```python
from build123d import *

# Parameters (mm, degrees)
EXTRUDE_1_DEPTH     = 4
CUT_EXTRUDE_1_DEPTH = 1
FILLET_1_R          = 1
EXTRUDE_2_DEPTH     = 1


with BuildPart() as part:
    # 草图1 → 凸台-拉伸1 (new body)
    with BuildSketch(Plane(origin=(0, 0, 0), x_dir=(1, 0, 0), z_dir=(0, 1, 0))):
        Polygon((14.43375673, 0), (7.216878365, 12.5), (-7.216878365, 12.5), (-14.43375673, 0), (-7.216878365, -12.5), (7.216878365, -12.5), align=None)
    extrude(amount=EXTRUDE_1_DEPTH)

    # 草图2 → 切除-拉伸1 (cut)
    with BuildSketch(Plane(origin=(0, 4, 0), x_dir=(1, 0, 0), z_dir=(0, 1, 0))):
        Polygon((5.484827557, -9.5), (10.969655115, 0), (5.484827557, 9.5), (-5.484827557, 9.5), (-10.969655115, 0), (-5.484827557, -9.5), align=None)
    extrude(amount=-CUT_EXTRUDE_1_DEPTH, mode=Mode.SUBTRACT)

    # 圆角1
    fillet_1_edges = [part.edges().sort_by_distance(p)[0] for p in [
        (7.216878365, 2, 12.5),
        (-7.216878365, 2, 12.5),
        (-14.43375673, 2, 0),
        (-7.216878365, 2, -12.5),
        (7.216878365, 2, -12.5),
        (14.43375673, 2, 0),
        (5.484827557, 3.5, 9.5),
        (-5.484827557, 3.5, 9.5),
        (-10.969655115, 3.5, 0),
        (-5.484827557, 3.5, -9.5),
        (5.484827557, 3.5, -9.5),
        (10.969655115, 3.5, 0),
    ]]
    fillet(fillet_1_edges, radius=FILLET_1_R)

    # 草图3 → 凸台-拉伸2 (add)
    with BuildSketch(Plane(origin=(0, 3, 0), x_dir=(1, 0, 0), z_dir=(0, 1, 0))):
        Polygon((4.270525574, -2.13873515), (1.319973126, 3.653003816), (-1.5, 0), (-4.270525574, 2.13873515), (-1.319973126, -3.653003816), (1.5, 0), align=None)
        with BuildLine():
            Line((4.73426289, -3.650545759), (5.922130387, -4.566499256))
            ThreePointArc((5.922130387, -4.566499256), (-0.023704107, 7.478233875), (-5.893062385, -4.603950425))
            Line((-5.893062385, -4.603950425), (-4.71102538, -3.68048493))
            ThreePointArc((-4.71102538, -3.68048493), (-0.018949511, 5.978241411), (4.73426289, -3.650545759))
        make_face()
    extrude(amount=EXTRUDE_2_DEPTH)


solid = part.part
```
Check sheet for the modelled part. Datum: model origin and axes. Units: mm. A direction names the side the tool comes from. Give positions to 0.01 mm unless a question says otherwise; leave off trailing zeros. Write each loop counter-clockwise with the first axis right and the second up, starting at its lowest first coordinate (ties: lowest second). Pieces come first, ordered by that corner, then holes.
Item 1: Access from +Z, -Z, +X, -X, +Y, -Y to the whole of each face (thin tool, end or side, straight path). Record for faces 1 (the face through (0, 0, 0)), 2 (the face through (-0.206, 3.493, -5.975)).
Item 2: Cross-section at A-A (y = 3.4). Count the separate pieces of the cut face and the enclosed holes in it, and give its area (3 significant figures).
Item 3: Gauge pin test, flat ends, axial feed: pin 1 (2 mm diameter, centred on y = 1.5, z = 5.5, fed in from -X); pin 2 (1 mm diameter, centred on y = 0.5, z = 3, fed in from -X). Record the tip position at first contact, or that the pin passes through.
Item 4: Cross-section at C-C (z = -8.25). Enter the section's corners in (x, y).
Item 5: Cross-section at D-D (x = 9). Enter the section's corners in (y, z).
Item 6: Draft check along Z on faces 3 (the face through (2.866, 3.493, 1.054)), 4 (the face through (10.78, 1.97, 6.33)), 5 (the face through (0, 4, 0)). Enter one of: released by +Z, released by -Z, zero draft, split by the parting line, or undercut.
Item 7: Scan lines: L1, parallel to Z at x = 0, y = 3.75; L2, parallel to Z at x = 6.5, y = 3.2; L3, parallel to Z at x = 2.5, y = 3.7. Record each from-to range of solid material in increasing order.
Item 8: Cross-section at B-B (y = 1.3). Enter the section's corners in (x, z).
Report:
1. face 1: +Z, -Z, +X, -X, -Y
1. face 2: +Y
2. separate pieces: 3
2. enclosed holes: 1
2. area: 294 mm2
3. pin 1: stops at x = -11.84
3. pin 2: stops at x = -12.99
4. outline: (-9.67, 0) - (9.67, 0) - (9.67, 4) - (6.21, 4) - (6.21, 3) - (-6.21, 3) - (-6.21, 4) - (-9.67, 4) - close
5. outline: (0, -9.41) - (4, -9.41) - (4, -3.41) - (3, -3.41) - (3, 3.41) - (4, 3.41) - (4, 9.41) - (0, 9.41) - close
6. face 3: undercut
6. face 4: released by +Z
6. face 5: zero draft
7. L1: z = -12.5 to -9.5, -7.48 to -5.98, -1.94 to 1.94, 9.5 to 12.5
7. L2: z = -12.5 to -7.74, -3.7 to 3.7, 7.74 to 12.5
7. L3: z = -12.5 to -9.5, -7.05 to -5.43, -1.34 to 0.77, 9.5 to 12.5
8. outline: (-14.15, -0.5) - (-7.51, -12) arc R1 ccw to (-6.64, -12.5) - (6.64, -12.5) arc R1 ccw to (7.51, -12) - (14.15, -0.5) arc R1 ccw to (14.15, 0.5) - (7.51, 12) arc R1 ccw to (6.64, 12.5) - (-6.64, 12.5) arc R1 ccw to (-7.51, 12) - (-14.15, 0.5) arc R1 ccw to start
